Input: part model. Units: mm. Frame: model coordinates. A direction names the side the tool comes from. Round coordinates to 2 decimals unless told otherwise and drop trailing zeros. Loops run counter-clockwise (first coordinate to the right, second up) from the corner with the lowest first, then second, coordinate; pieces in that order, holes last. Notation, with made-up numbers: (19.25, 27.5) -> (29.25, 27.5) arc R20 ccw to (29.25, 36.5) -> close; hole circle Ø8 at (11.5, 8). An arc over 180 degrees is marked (long way). Answer as a JSON object with one key per item and string values. Group by question number.
Item 1: Material intervals for line 1 (Y direction, x = -94, z = 1.95); line 2 (Y direction, x = -170, z = 3.4); line 3 (X direction, y = 8.5, z = 3.35), sorted ascending. Write a range as [from, to].
Item 2: Set-up query: faces 4 (the flat face through (-117, 11.564, 2)), 5 (the flat face through (12.44, -40.65, 2.54)), 6 (the flat face through (-147, -66, 2)). Return all of +Z, -Z, +X, -X, +Y, -Y with unobstructed straight access to the full face (end or side cutting, diameter ignored); none if empty.
Item 3: Draft query along Y for faces 1 (the cylindrical face through (-36.938, 15.496, 2.465)), 2 (the cylindrical face through (-28.504, 3.083, 2.535)), 3 (the cylindrical face through (-8.013, -91.17, 2.465)). Return one class per face: released by +Y, released by -Y, zero draft, split by the parting line, or undercut.
Item 4: Section query A-A on x = -110. Return loops of the section in (y, z), and give its area (3 significant figures).
Item 5: Section query C-C on z = 3.6. Return loops of the section in (x, y).
Item 6: Section query B-B on y = 28.5. Return loops of the section in (x, z).
Item 7: Pin query (flat end, axial travel): pin 1 (2.5 mm diameter, centred on x = -169, z = 3, fed in from +Y); pin 2 (3 mm diameter, centred on y = -75, z = 4, fed in from +X); pin 3 (2.5 mm diameter, centred on y = -69, z = 3.5, fed in from -X). Return the tip coordinate at first contact, or that it passes through.
Autodesk Inventor part; units mm, degrees
ref_plane "YZ Plane" through (0, 0, 0) normal (1, 0, 0) x (0, 1, 0)
ref_plane "XZ Plane" through (0, 0, 0) normal (0, 1, 0) x (-1, 0, 0)
ref_plane "XY Plane" through (0, 0, 0) normal (0, 0, 1) x (1, 0, 0)
sketch "Sketch1" plane through (0, 0, 0) normal (0, 0, 1) x (1, 0, 0)
  line L0 (-48.8466, 11.5644) -> (-187, 11.5644)
  line L1 (-187, 11.5644) -> (-187, -38.4356)
  line L2 (-187, -38.4356) -> (-167, -38.4356)
  line L3 (-147, -58.4356) -> (-147, -73.4356)
  line L4 (-127, -93.4356) -> (-17.2605, -93.4356)
  arc A0 (49.5519, -14.6836) -> (-29.8169, 25.4105) centre (13, 11.5644) ccw
  line L5 (49.5519, -14.6836) -> (-1.0152, -85.1014)
  arc A1 (-48.8466, 11.5644) -> (-29.8169, 25.4105) centre (-48.8466, 31.5644) ccw
  arc A2 (-147, -58.4356) -> (-167, -38.4356) centre (-167, -58.4356) ccw
  arc A3 (-147, -73.4356) -> (-127, -93.4356) centre (-127, -73.4356) ccw
  arc A4 (-17.2605, -93.4356) -> (-1.0152, -85.1014) centre (-17.2605, -73.4356) ccw
  point P0 (0, 0)
  point P1 (-32, 11.5644)
  point P2 (-147, -38.4356)
  point P3 (-147, -93.4356)
  point P4 (-7, -93.4356)
  dimension "d1" = 0
  dimension "d2" = 105
  dimension "d21" = 200
  dimension "d22" = 40
  dimension "d23" = 50
  dimension "d24" = 180
  dimension "d25" = 45
  dimension "d38" = 20
  dimension "d39" = 20
extrude "Extrusion1" add sketch "Sketch1" along normal blind 5
sketch "Sketch2" plane through (0, 0, 5) normal (0, 0, 1) x (1, 0, 0)
  arc A0 (-48.8466, 11.5644) -> (-29.8169, 25.4105) centre (-48.8466, 31.5644) ccw
  line L0 (-48.8466, 11.5644) -> (-187, 11.5644)
  line L1 (-187, 11.5644) -> (-187, -38.4356)
  line L2 (-187, -38.4356) -> (-167, -38.4356)
  arc A1 (-147, -58.4356) -> (-167, -38.4356) centre (-167, -58.4356) ccw
  line L3 (-147, -58.4356) -> (-147, -73.4356)
  arc A2 (-147, -73.4356) -> (-127, -93.4356) centre (-127, -73.4356) ccw
  line L4 (-127, -93.4356) -> (-17.2605, -93.4356)
  arc A3 (-17.2605, -93.4356) -> (-1.0152, -85.1014) centre (-17.2605, -73.4356) ccw
  line L5 (-1.0152, -85.1014) -> (49.5519, -14.6836)
  arc A4 (49.5519, -14.6836) -> (-29.8169, 25.4105) centre (13, 11.5644) ccw
  line L6 (-172, -3.4356) -> (-48.8466, -3.4356)
  arc A5 (-48.8466, -3.4356) -> (-15.5446, 20.7951) centre (-48.8466, 31.5644) ccw
  arc A6 (37.368, -5.9343) -> (-15.5446, 20.7951) centre (13, 11.5644) ccw
  line L7 (37.368, -5.9343) -> (-13.1992, -76.3521)
  arc A7 (-17.2605, -78.4356) -> (-13.1992, -76.3521) centre (-17.2605, -73.4356) ccw
  line L8 (-17.2605, -78.4356) -> (-127, -78.4356)
  arc A8 (-132, -73.4356) -> (-127, -78.4356) centre (-127, -73.4356) ccw
  line L9 (-132, -73.4356) -> (-132, -58.4356)
  arc A9 (-132, -58.4356) -> (-167, -23.4356) centre (-167, -58.4356) ccw
  line L10 (-167, -23.4356) -> (-172, -23.4356)
  line L11 (-172, -23.4356) -> (-172, -3.4356)
  point P0 (0, 0)
  dimension "d42" = 15
extrude "Extrusion2" cut sketch "Sketch2" against normal through all contours L6 A5 A6 L7 A7 L8 A8 L9 A9 L10 L11
sketch "Sketch3" plane through (0, 0, 5) normal (0, 0, 1) x (1, 0, 0)
  point P0 (0, 0)
sketch "Sketch4" plane through (0, 0, 5) normal (0, 0, 1) x (1, 0, 0)
  point P0 (0, 0)
properties part number "GASKET"
Solved:
{
 "1": {"line 1": "[-93.44, -78.44], [-3.44, 11.56]", "line 2": "[-38.44, -23.44], [-3.44, 11.56]", "line 3": "[-187, -22.52], [42.84, 57.9]"},
 "2": {"face 4": "+Z, -Z, -X, +Y", "face 5": "+Z, -Z", "face 6": "+Z, -Z, -X, -Y"},
 "3": {"face 1": "released by +Y", "face 2": "undercut", "face 3": "released by -Y"},
 "4": {"outline": "(-93.44, 0) -> (-78.44, 0) -> (-78.44, 5) -> (-93.44, 5) -> close; (-3.44, 0) -> (11.56, 0) -> (11.56, 5) -> (-3.44, 5) -> close", "area": "150 mm²"},
 "5": {"outline": "(-187, -38.44) -> (-167, -38.44) arc R20 cw to (-147, -58.44) -> (-147, -73.44) arc R20 ccw to (-127, -93.44) -> (-17.26, -93.44) arc R20 ccw to (-1.02, -85.1) -> (49.55, -14.68) arc R45 ccw (long way) to (-29.82, 25.41) arc R20 cw to (-48.85, 11.56) -> (-187, 11.56) -> close; hole (-172, -23.44) -> (-167, -23.44) arc R35 cw to (-132, -58.44) -> (-132, -73.44) arc R5 ccw to (-127, -78.44) -> (-17.26, -78.44) arc R5 ccw to (-13.2, -76.35) -> (37.37, -5.93) arc R30 ccw (long way) to (-15.54, 20.8) arc R35 cw to (-48.85, -3.44) -> (-172, -3.44) -> close"},
 "6": {"outline": "(-28.69, 0) -> (-11.76, 0) -> (-11.76, 5) -> (-28.69, 5) -> close; (37.76, 0) -> (54.69, 0) -> (54.69, 5) -> (37.76, 5) -> close"},
 "7": {"pin 1": "y = 11.56", "pin 2": "x = 7.32", "pin 3": "x = -147"}
}
